Build history of the part. All positions in model axes, mm. Round coordinates to 2 decimals unless told otherwise and drop trailing zeros. Write each loop counter-clockwise with the first axis right and the second up, starting at its lowest first coordinate (ties: lowest second). Pieces come first, ordered by that corner, then holes. Notation, with made-up numbers: M 22,-22.75 L 77,-22.75 A31 ccw 77,1.25 Z; hole C 11,82 d2. An arc over 180 degrees is marked long. Write item = value, one per line.
Autodesk Inventor part; units mm, degrees
ref_plane "YZ Plane" through (0, 0, 0) normal (1, 0, 0) x (0, 1, 0)
ref_plane "XZ Plane" through (0, 0, 0) normal (0, 1, 0) x (-1, 0, 0)
ref_plane "XY Plane" through (0, 0, 0) normal (0, 0, 1) x (1, 0, 0)
sketch "Sketch1" plane through (0, 0, 0) normal (0, 0, 1) x (1, 0, 0)
  line L0 (-11.1101, 6.0966) -> (-9.5601, 3.3251)
  line L1 (-9.5601, 3.3251) -> (-11.1853, 0.5971)
  line L2 (-11.1853, 0.5971) -> (-14.3604, 0.6405)
  line L3 (-14.3604, 0.6405) -> (-15.9104, 3.412)
  line L4 (-15.9104, 3.412) -> (-14.2852, 6.14)
  line L5 (-14.2852, 6.14) -> (-11.1101, 6.0966)
  circle A0 centre (-12.7353, 3.3685) radius 1.5
  dimension "d0" = 5.5
  dimension "d1" = 3
extrude "Extrusion1" add sketch "Sketch1" along normal blind 10
thread "Thread2"
thread "Thread3"
properties part number "Espaciador para Electrónica 10mm" material "Acetal Resin, White"
1. Mould opens along Y. For faces 1 (the face through (-10.346, 4.73, 4.93)), 2 (the face through (-11, 4, 10)), 3 (the face through (-11.35, 3.94, 4.93)) say: pulls with the +Y half, pulls with the -Y half, needs draft (parallel to the pull), parting line crosses it, or undercut.
Responses:
face_1 = pulls with the +Y half
face_2 = needs draft
face_3 = undercut
2. Band-saw the part on B-B (x = -12.5). List the corners of the cut face in (y, z).
Responses:
outline = M 0.62,0 L 1.89,0 L 1.89,10 L 0.62,10 Z; M 4.85,0 L 6.12,0 L 6.12,10 L 4.85,10 Z
3. Band-saw the part on D-D (x = -10). List the corners of the cut face in (y, z).
Responses:
outline = M 2.59,0 L 4.11,0 L 4.11,10 L 2.59,10 Z
4. Probe probe 1 along Y at (x, z) = (-11.75, 5.25); probe 2 along X at (y, z) = (4.1, 4.25); probe 3 along Y at (x, z) = (-12.5, 1.5). List the from-to ranges inside material, lowest first.
Responses:
probe_1 = 0.6 to 2.24, 4.5 to 6.11
probe_2 = -15.5 to -14.04, -11.43 to -9.99
probe_3 = 0.62 to 1.89, 4.85 to 6.12
5. Band-saw the part on A-A (y = 4.7). List the corners of the cut face in (x, z), plus the area to 3 significant figures.
Responses:
outline = M -15.14,0 L -13.43,0 L -13.43,10 L -15.14,10 Z; M -12.04,0 L -10.33,0 L -10.33,10 L -12.04,10 Z
area = 34.3 mm²
6. Flat gauge pins, fed straight in: pin 1 (3 mm diameter, centred on x = -12.5, z = 6.5, fed in from -Y); pin 2 (2 mm diameter, centred on x = -11.5, z = 3, fed in from +Y). Where does each tip first touch, or does it go through?
Responses:
pin_1 = 0.6
pin_2 = 6.12
7. Band-saw the part on C-C (z = 1.5). List the corners of the cut face in (x, y).
Responses:
outline = M -15.91,3.41 L -14.36,0.64 L -11.19,0.6 L -9.56,3.33 L -11.11,6.1 L -14.29,6.14 Z; hole C -12.74,3.37 d3
